The listing builds one solid part. Answer for the finished solid, in the listing's coordinates (mm). Face numbers are marked on the shaded views. A direction names the side the tool comes from. Give positions to 0.01 mm unless a question says otherwise; leave off trailing zeros. Order: outer loops, then holes, each group sorted by start corner. A loop starts at its lowest first (then second) coordinate and runs counter-clockwise, first axis right, second up. Notation, with made-up numbers: (78.25, 31) - (88.25, 31) arc R16 cw to (88.25, 39) - close; hole circle Ø8 at (27.5, 61). An arc over 180 degrees is marked (long way). Answer in a Markdown table with one row per item.
from build123d import *

# Parameters (mm, degrees)
SKETCH_1_W          = 20.2
SKETCH_1_H          = 15.4
EXTRUDE_1_DEPTH     = 25
SKETCH_2_R          = 2.5
EXTRUDE_2_DEPTH     = 1.5
SKETCH_3_R          = 1
EXTRUDE_3_DEPTH     = 10
FILLET_2_SIZE       = 7.7
FILLET_2_SIZE_2     = 4
FILLET_3_SIZE       = 4
FILLET_3_SIZE_2     = 7.7
SKETCH_4_R          = 1
CUT_EXTRUDE_1_DEPTH = 5
SKETCH_5_R          = 2.5
EXTRUDE_4_DEPTH     = 1.5
SKETCH_6_W          = 0.2
SKETCH_6_H          = 3
EXTRUDE_5_DEPTH     = 4
FILLET_4_R          = 1
SKETCH_7_R          = 0.3
CUT_EXTRUDE_2_DEPTH = 44.016597153


with BuildPart() as part:
    # 草图1 → 凸台-拉伸1 (new body)
    with BuildSketch(Plane.XY):
        with Locations((10.1, -7.7)):
            Rectangle(SKETCH_1_W, SKETCH_1_H)
    extrude(amount=EXTRUDE_1_DEPTH)

    # 草图2 → 凸台-拉伸2 (add)
    with BuildSketch(Plane.XY.offset(25)):
        with Locations((10.2, -7.5)):
            Circle(SKETCH_2_R)
    extrude(amount=EXTRUDE_2_DEPTH)

    # 草图3 → 凸台-拉伸3 (add)
    with BuildSketch(Plane.XY.offset(26.5)):
        with Locations((10.2, -7.5)):
            Circle(SKETCH_3_R)
    extrude(amount=EXTRUDE_3_DEPTH)

    # 圆角2
    # an asymmetric fillet: 7.7, 4 mm, written as the material it takes off along each edge
    with BuildSketch(Plane(origin=(20.2, -15.4, -19.25), x_dir=(0, 1, 0), z_dir=(0, 0, 1))) as fillet_2_piece_1:
        with BuildLine():
            Bezier((FILLET_2_SIZE, 0), (0, 0), (0, FILLET_2_SIZE_2), weights=[1, 0.707106781, 1])
            Line((0, FILLET_2_SIZE_2), (0, 0))
            Line((0, 0), (FILLET_2_SIZE, 0))
        make_face()
    extrude(amount=63.5, mode=Mode.SUBTRACT)
    with BuildSketch(Plane(origin=(0, 0, -19.25), x_dir=(1, 0, 0), z_dir=(0, 0, 1))) as fillet_2_piece_2:
        with BuildLine():
            Bezier((FILLET_2_SIZE_2, 0), (0, 0), (0, -FILLET_2_SIZE), weights=[1, 0.707106781, 1])
            Line((0, -FILLET_2_SIZE), (0, 0))
            Line((0, 0), (FILLET_2_SIZE_2, 0))
        make_face()
    extrude(amount=63.5, mode=Mode.SUBTRACT)

    # 圆角3
    # an asymmetric fillet: 7.7, 4 mm, written as the material it takes off along each edge
    with BuildSketch(Plane(origin=(20.2, 0, -19.25), x_dir=(-1, 0, 0), z_dir=(0, 0, 1)), Plane(origin=(0, -15.4, -19.25), x_dir=(1, 0, 0), z_dir=(0, 0, 1))) as fillet_3_piece_1:
        with BuildLine():
            Bezier((FILLET_3_SIZE, 0), (0, 0), (0, FILLET_3_SIZE_2), weights=[1, 0.707106781, 1])
            Line((0, FILLET_3_SIZE_2), (0, 0))
            Line((0, 0), (FILLET_3_SIZE, 0))
        make_face()
    extrude(amount=63.5, mode=Mode.SUBTRACT)

    # 草图4 → 切除-拉伸1 (cut)
    with BuildSketch(Plane.XY.offset(25)):
        with Locations((3.95, -7.7)):
            Circle(SKETCH_4_R)
        with Locations((16.45, -7.7)):
            Circle(SKETCH_4_R)
    extrude(amount=-CUT_EXTRUDE_1_DEPTH, mode=Mode.SUBTRACT)

    # 草图5 → 凸台-拉伸4 (add)
    with BuildSketch(Plane(origin=(0, 0, 0), x_dir=(-1, 0, 0), z_dir=(0, 0, -1))):
        with Locations(Location((-10.1, -7.7, 0), (0, 0, 180))):
            Circle(SKETCH_5_R)
    extrude(amount=EXTRUDE_4_DEPTH)

    # 草图6 → 凸台-拉伸5 (add)
    with BuildSketch(Plane(origin=(0, 0, 0), x_dir=(-1, 0, 0), z_dir=(0, 0, -1))):
        with Locations((-3.536419709, -7.7)):
            Rectangle(SKETCH_6_W, SKETCH_6_H)
        with Locations((-16.302368295, -7.7)):
            Rectangle(SKETCH_6_W, SKETCH_6_H)
    extrude(amount=EXTRUDE_5_DEPTH)

    # 圆角4
    fillet_4_edges = [part.edges().sort_by_distance(p)[0] for p in [
        (3.536419709, -6.2, -4),
        (3.536419709, -9.2, -4),
        (16.302368295, -6.2, -4),
        (16.302368295, -9.2, -4),
    ]]
    fillet(fillet_4_edges, radius=FILLET_4_R)

    # 草图7 → 切除-拉伸2 (cut, through all)
    with BuildSketch(Plane.ZY.offset(-3.436419709)):
        with Locations((-3, -7.7)):
            Circle(SKETCH_7_R)
    extrude(amount=-CUT_EXTRUDE_2_DEPTH, mode=Mode.SUBTRACT)


solid = part.part
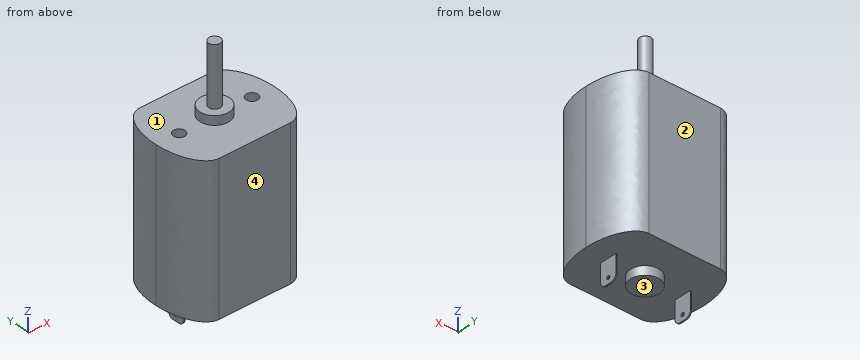
Item 1: Find section A-A on x = 10.1. Write down the section's boundary in (y, z).
Answer block:
| item | result |
|---|---|
| outline | (-15.4, 0) - (-10.2, 0) - (-10.2, -1.5) - (-5.2, -1.5) - (-5.2, 0) - (0, 0) - (0, 25) - (-5, 25) - (-5, 26.5) - (-6.51, 26.5) - (-6.51, 36.5) - (-8.49, 36.5) - (-8.49, 26.5) - (-10, 26.5) - (-10, 25) - (-15.4, 25) - close |
Item 2: Consider line 1 (Y direction, x = 3.55, z = -3); line 2 (Z direction, x = 3, y = -6); line 3 (Y direction, x = 10.25, z = -1). Determine where each line is inside the solid, lowest interval first.
Answer block:
| item | result |
|---|---|
| line 1 | -9.2 to -8, -7.4 to -6.2 |
| line 2 | 0 to 25 |
| line 3 | -10.2 to -5.2 |
Item 3: Each of these flat-tipped pins is pushed along its axis until it touches: P1, Ø1.5, axis at y = -7.5, z = -1.5, coming from the +X side; P2, Ø5, axis at x = 7.5, y = -10, coming from the -Z side; P3, Ø2, axis at x = 17, y = -1.5, coming from the +Z side. Where does it stop, or does it pass through?
Answer block:
| item | result |
|---|---|
| P1 | x = 16.4 |
| P2 | z = -1.5 |
| P3 | z = 25 |
Item 4: Which of the six approach directions +Z, -Z, +X, -X, +Y, -Y give full straight-line access (tool end or side, diameter ignored) to the marked faces 1 and 2?
Answer block:
| item | result |
|---|---|
| face 1 | +Z |
| face 2 | +Z, -Z, +X, -X, +Y |
Item 5: Determine the mould class of the marked faces 3 and 4 for opening direction X: pulls with the +X half, pulls with the -X half, needs draft (parallel to the pull), parting line crosses it, or undercut.
Answer block:
| item | result |
|---|---|
| face 3 | undercut |
| face 4 | needs draft |
Item 6: Find section C-C on x = 14.5. Write down the section's boundary in (y, z).
Answer block:
| item | result |
|---|---|
| outline | (-15.4, 0) - (0, 0) - (0, 25) - (-15.4, 25) - close |
Item 7: Find section B-B on z = 29. Write down the section's boundary in (x, y).
Answer block:
| item | result |
|---|---|
| outline | circle Ø2 at (10.2, -7.5) |
